Work out the finished part from the listing and answer in its coordinate system (mm). A direction names the side the tool comes from. Coordinates: 2 decimals unless noted, no trailing zeros. Order: outer loops, then holes, each group sorted by start corner. A loop starts at its lowest first (then second) coordinate and runs counter-clockwise, first axis right, second up. Notation, with made-up numbers: (-6, 18) - (21, 18) arc R22 ccw to (21, 42) - close; hole circle Ø9 at (48.5, 24). An arc over 180 degrees is marked (long way). Use CSV: the item, a comma, the result in double quotes. Start each with the question number.
from build123d import *

# Parameters (mm, degrees)
F0_W     = 160
F0_H     = 74
F1_DEPTH = 12
F0_H_2   = 8
F2_DEPTH = 20


with BuildPart() as f1:
    # F0 (on Right) → F1 (new body)
    with BuildSketch(Plane.YZ):
        Polygon((-73.062379, 19.760398), (-93.062379, 19.760398), (-93.062379, -70.239602), (106.937621, -70.239602), (106.937621, 19.760398), (86.937621, 19.760398), (86.937621, 11.760398), (-73.062379, 11.760398), align=None)
        with Locations((6.937621, -29.239602)):
            Rectangle(F0_W, F0_H, mode=Mode.SUBTRACT)
    extrude(amount=F1_DEPTH)

    # F0 (on Right) → F2 (join)
    with BuildSketch(Plane.YZ):
        with Locations((6.937621, 15.760398)):
            Rectangle(F0_W, F0_H_2)
        with Locations((6.937621, -29.239602)):
            Rectangle(F0_W, F0_H)
    extrude(amount=F2_DEPTH)


solid = f1.part
1) The part is cut by section B-B on z = -28.5. Determine the outline of the cut face in (x, y).
2) Straight lines are drawn through the part: line 1 (Z direction, x = 15.5, y = -68); line 2 (Y direction, x = 13.5, z = -13.5); line 3 (X direction, y = -84, z = -22.5). For each, find the intervals that lie inside material, in ascending order. Write a range as [from, to].
3) The part is cut by section A-A on y = -3.5. Determine the outline of the cut face in (x, z), plus the area to 3 significant figures.
4) Flat-ended cylindrical pins translate along their axes: P1, Ø1.5, axis at x = 13, y = -0.5, coming from the -Z side; P2, Ø2.5, axis at x = 16, z = -12.5, coming from the +Y side; P3, Ø4, axis at x = 17.5, z = 17, coming from the -Y side. Find the tip coordinate at first contact, or state that the pin passes through.
5) For faces 5 (the face through (16, 86.938, -30)), 6 (the face through (16, 6, 11.76)), 7 (the face through (16, -73.062, 16)), determine the directions among +Z, -Z, +X, -X, +Y, -Y from which every point of the face is accessible in a straight line to the end or side of a thin tool.
6) For a pull along Z with two mould halves and no side action, classify faces 1 (the face through (16, 6, 7.76)), 2 (the face through (12, 14, 8)), 3 (the face through (20, 6, -29)), 4 (the face through (10, 6, 19.76)) as +Z half, -Z half, draft (parallel to the pull), parting line (faces both ways), or undercut.
Answer key:
1,outline,"(0, -93.06) - (12, -93.06) - (12, -73.06) - (20, -73.06) - (20, 86.94) - (12, 86.94) - (12, 106.94) - (0, 106.94) - close"
2,line 1,"[-66.24, 7.76], [11.76, 19.76]"
2,line 2,"[-73.06, 86.94]"
2,line 3,"[0, 12]"
3,outline,"(0, -70.24) - (12, -70.24) - (12, -66.24) - (20, -66.24) - (20, 7.76) - (12, 7.76) - (12, 11.76) - (20, 11.76) - (20, 19.76) - (0, 19.76) - close"
3,area,"1,740 mm^2"
4,P1,"z = -66.24"
4,P2,"y = 86.94"
4,P3,"y = -73.06"
5,face 5,"+Z, -Z, +X, +Y"
5,face 6,"+X, +Y, -Y"
5,face 7,"+Z, -Z, +X, -Y"
6,face 1,"undercut"
6,face 2,"undercut"
6,face 3,"draft"
6,face 4,"+Z half"
